Can you work these out from the model? Positions are in its coordinate system, mm. Face numbers are marked on the shaded views. A direction names the side the tool comes from. Round coordinates to 2 decimals unless told otherwise and drop trailing zeros. Write each loop counter-clockwise with the first axis right and the second up, starting at its lowest first coordinate (ties: lowest second). Pieces come first, ordered by that corner, then holes. Notation, with made-up numbers: (-13, 27.5) -> (17, 27.5) arc R13 cw to (17, 43.5) -> close; hole circle Ø1 at (-9.75, 58). An arc over 180 degrees is marked (long way). Write item = value, one per line. Start each with the question number.
1) I'm going to push flat-ended pins straight in: pin 1 (5 mm diameter, centred on y = 8.8, z = -53.6, fed in from -X); pin 2 (8 mm diameter, centred on x = -86, y = 8, fed in from -Z); pin 3 (2.5 mm diameter, centred on y = 34.5, z = -53.6, fed in from +X). Where does each tip first touch, or does it pass through?
2) If I drill on line 1 (Z direction, x = -7, y = 0.8); line 2 (Z direction, x = -66, y = 28); line 3 (X direction, y = 0.5, z = -90.6), over which ranges is the centre line in solid material (lowest first)?
3) Imagine slicing it at B-B, the plane z = -53.6. Please give me the cut outline in (x, y), then the cut area to 3 significant figures.
4) Thinking about a two-plate mould opening in Z: for the marked faces 3, 4 and 5, which applies, +Z half, -Z half, draft (parallel to the pull), parting line (faces both ways), or undercut?
5) Imagine slicing it at D-D, the plane x = -34. Please give me the cut outline in (y, z).
6) For the marked faces 1 and 2, which set-ups out of +Z, -Z, +X, -X, +Y, -Y let a thin tool reach every point of the face, with its end or its side?
7) Imagine slicing it at A-A, the plane z = -90.6. Please give me the cut outline in (x, y).
8) Imagine slicing it at C-C, the plane y = 8.8. State how many separate pieces and enclosed holes the cut face has, then the cut area to 3 significant figures.
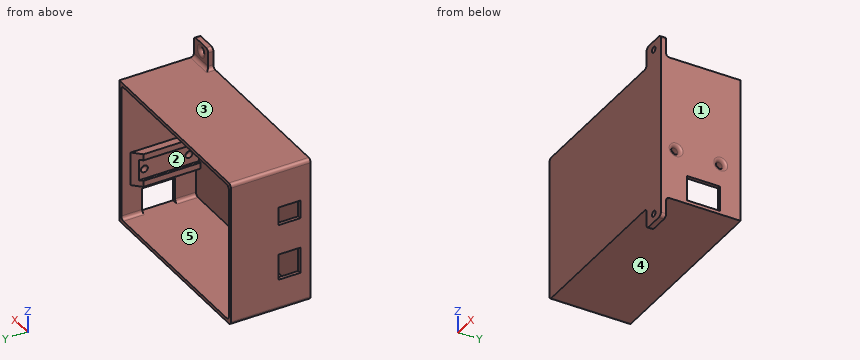
from build123d import *

# Parameters (mm, degrees)
BOSS_EXTRUDE1_DEPTH = 46
BOSS_EXTRUDE2_DEPTH = 3
BOSS_EXTRUDE3_DEPTH = 3
FILLET1_R           = 2
FILLET2_R           = 2
CUT_EXTRUDE5_REACH  = 154.825
SKETCH3_R           = 1.7
FILLET3_R           = 2
CUT_EXTRUDE6_DEPTH  = 43
SKETCH5_W           = 4.6
SKETCH5_H           = 19.4
BOSS_EXTRUDE4_DEPTH = 46
SKETCH6_W           = 4.6
SKETCH6_H           = 19.4
CUT_EXTRUDE8_DEPTH  = 5
SKETCH7_W           = 1.6
SKETCH7_H           = 12.2
CUT_EXTRUDE10_DEPTH = 38
CHAMFER1_SIZE       = 5
SKETCH8_R           = 2
CUT_EXTRUDE11_DEPTH = 34.5
FILLET4_R           = 2
SKETCH12_W          = 15
SKETCH12_H          = 12.6
SKETCH12_W_2        = 10.5
CUT_EXTRUDE13_DEPTH = 34.5
SKETCH14_W          = 14.5
SKETCH14_H          = 19
CUT_EXTRUDE14_DEPTH = 10


with BuildPart() as part:
    # Sketch2 → Boss-Extrude1 (new body)
    with BuildSketch(Plane(origin=(0, 0, 0), x_dir=(1, 0, 0), z_dir=(0, 1, 0))):
        with BuildLine():
            ThreePointArc((-110, 81.6), (-109.414213562, 83.014213562), (-108, 83.6))
            Line((-108, 83.6), (-16, 83.6))
            Line((-16, 83.6), (0, 83.6))
            Line((0, 83.6), (0, 0))
            Line((0, 0), (-16, 0))
            Line((-16, 0), (-108, 0))
            ThreePointArc((-108, 0), (-109.414213562, 0.585786438), (-110, 2))
            Line((-110, 2), (-110, 81.6))
        make_face()
    extrude(amount=BOSS_EXTRUDE1_DEPTH)

    # Sketch2<7> → Boss-Extrude2 (add)
    with BuildSketch(Plane(origin=(0, 0, 0), x_dir=(1, 0, 0), z_dir=(0, 1, 0))):
        with BuildLine():
            ThreePointArc((-16, 83.6), (-14.585786438, 84.185786438), (-14, 85.6))
            Line((-14, 85.6), (-14, 93.6))
            ThreePointArc((-14, 93.6), (-13.414213562, 95.014213562), (-12, 95.6))
            Line((-12, 95.6), (-2, 95.6))
            ThreePointArc((-2, 95.6), (-0.585786438, 95.014213562), (0, 93.6))
            Line((0, 93.6), (0, 83.6))
            Line((0, 83.6), (-16, 83.6))
        make_face()
    extrude(amount=BOSS_EXTRUDE2_DEPTH)

    # Sketch2<8> → Boss-Extrude3 (add)
    with BuildSketch(Plane(origin=(0, 0, 0), x_dir=(1, 0, 0), z_dir=(0, 1, 0))):
        with BuildLine():
            ThreePointArc((0, -10), (-0.585786438, -11.414213562), (-2, -12))
            Line((-2, -12), (-12, -12))
            ThreePointArc((-12, -12), (-13.414213562, -11.414213562), (-14, -10))
            Line((-14, -10), (-14, -2))
            ThreePointArc((-14, -2), (-14.585786438, -0.585786438), (-16, 0))
            Line((-16, 0), (0, 0))
            Line((0, 0), (0, -10))
        make_face()
    extrude(amount=BOSS_EXTRUDE3_DEPTH)

    # Fillet1
    fillet1_edges = [part.edges().sort_by_distance(p)[0] for p in [
        (-8, 3, -83.6),
    ]]
    fillet(fillet1_edges, radius=FILLET1_R)

    # Fillet2
    fillet2_edges = [part.edges().sort_by_distance(p)[0] for p in [
        (-8, 3, 0),
    ]]
    fillet(fillet2_edges, radius=FILLET2_R)

    # Sketch3 → Cut-Extrude5 (cut, up to next)
    with BuildSketch(Plane(origin=(0, 0, 0), x_dir=(1, 0, 0), z_dir=(0, 1, 0)), mode=Mode.PRIVATE) as cut_extrude5_sk1:
        with Locations(Location((-7, -7, 0), (0, 0, 270))):
            Circle(SKETCH3_R)
    cut_extrude5_tool1 = extrude(cut_extrude5_sk1.sketch, amount=CUT_EXTRUDE5_REACH, mode=Mode.PRIVATE) & part.part
    # Sketch3 → Cut-Extrude5 (cut, up to next)
    with BuildSketch(Plane(origin=(0, 0, 0), x_dir=(1, 0, 0), z_dir=(0, 1, 0)), mode=Mode.PRIVATE) as cut_extrude5_sk2:
        with Locations(Location((-7, 90.6, 0), (0, 0, 270))):
            Circle(SKETCH3_R)
    cut_extrude5_tool2 = extrude(cut_extrude5_sk2.sketch, amount=CUT_EXTRUDE5_REACH, mode=Mode.PRIVATE) & part.part
    add(cut_extrude5_tool1.solids().sort_by_distance((-7, 0, 7))[0], mode=Mode.SUBTRACT)
    add(cut_extrude5_tool2.solids().sort_by_distance((-7, 0, -90.6))[0], mode=Mode.SUBTRACT)

    # Fillet3
    fillet3_edges = [part.edges().sort_by_distance(p)[0] for p in [
        (-7, 3, -92.3),
        (-7, 3, 5.3),
    ]]
    fillet(fillet3_edges, radius=FILLET3_R)

    # Sketch4 → Cut-Extrude6 (cut)
    with BuildSketch(Plane(origin=(0, 46, 0), x_dir=(1, 0, 0), z_dir=(0, 1, 0))):
        with BuildLine():
            Line((-106, 81.6), (-4, 81.6))
            ThreePointArc((-4, 81.6), (-2.585786438, 81.014213562), (-2, 79.6))
            Line((-2, 79.6), (-2, 4))
            ThreePointArc((-2, 4), (-2.585786438, 2.585786438), (-4, 2))
            Line((-4, 2), (-106, 2))
            ThreePointArc((-106, 2), (-107.414213562, 2.585786438), (-108, 4))
            Line((-108, 4), (-108, 79.6))
            ThreePointArc((-108, 79.6), (-107.414213562, 81.014213562), (-106, 81.6))
        make_face()
    extrude(amount=-CUT_EXTRUDE6_DEPTH, mode=Mode.SUBTRACT)

    # Sketch5 → Boss-Extrude4 (add)
    with BuildSketch(Plane(origin=(0, 0, 0), x_dir=(1, 0, 0), z_dir=(0, 1, 0))):
        with Locations((-4.3, 53.3)):
            Rectangle(SKETCH5_W, SKETCH5_H)
    extrude(amount=BOSS_EXTRUDE4_DEPTH)

    # Sketch6 → Cut-Extrude8 (cut)
    with BuildSketch(Plane(origin=(0, 46, 0), x_dir=(1, 0, 0), z_dir=(0, 1, 0))):
        with Locations((-4.3, 53.3)):
            Rectangle(SKETCH6_W, SKETCH6_H)
    extrude(amount=-CUT_EXTRUDE8_DEPTH, mode=Mode.SUBTRACT)

    # Sketch7 → Cut-Extrude10 (cut)
    with BuildSketch(Plane(origin=(0, 41, 0), x_dir=(1, 0, 0), z_dir=(0, 1, 0))):
        with Locations((-5.8, 53.3)):
            Rectangle(SKETCH7_W, SKETCH7_H)
    extrude(amount=-CUT_EXTRUDE10_DEPTH, mode=Mode.SUBTRACT)

    # Chamfer1
    # the kernel refuses this chamfer: 5 mm, written as the material it takes off along each edge
    with BuildSketch(Plane(origin=(-6.6, 41, -46.54158506), x_dir=(0.9996219169112968, 0.027495876610586317, 0), z_dir=(0, 0, -1))) as chamfer1_piece_1_section:
        Polygon((CHAMFER1_SIZE * 0.999621916911, CHAMFER1_SIZE * 0.0274958766106), (-CHAMFER1_SIZE * 0.0274958766106, CHAMFER1_SIZE * 0.999621916911), (0, 0), align=None)
    chamfer1_piece_1 = extrude(amount=29.31682988, mode=Mode.PRIVATE)
    chamfer1_piece_1 = split(chamfer1_piece_1, bisect_by=Plane(origin=(-2, 39.327890325, -61.2), z_dir=(-1, 0, 0)), keep=Keep.TOP, mode=Mode.PRIVATE)
    add(chamfer1_piece_1, mode=Mode.SUBTRACT)
    with BuildSketch(Plane(origin=(-6.6, 41, -30.74158506), x_dir=(0.9996219169112968, 0.027495876610586317, 0), z_dir=(0, 0, -1))) as chamfer1_piece_2_section:
        Polygon((CHAMFER1_SIZE * 0.999621916911, CHAMFER1_SIZE * 0.0274958766106), (-CHAMFER1_SIZE * 0.0274958766106, CHAMFER1_SIZE * 0.999621916911), (0, 0), align=None)
    chamfer1_piece_2 = extrude(amount=29.31682988, mode=Mode.PRIVATE)
    chamfer1_piece_2 = split(chamfer1_piece_2, bisect_by=Plane(origin=(-2, 39.327890325, -45.4), z_dir=(-1, 0, 0)), keep=Keep.TOP, mode=Mode.PRIVATE)
    add(chamfer1_piece_2, mode=Mode.SUBTRACT)

    # Sketch8 → Cut-Extrude11 (cut)
    with BuildSketch(Plane(origin=(0, 0, 0), x_dir=(0, 0, -1), z_dir=(1, 0, 0))):
        with Locations((53.6, 8.8)):
            Circle(SKETCH8_R)
        with Locations((53.6, 34.5)):
            Circle(SKETCH8_R)
    extrude(amount=-CUT_EXTRUDE11_DEPTH, mode=Mode.SUBTRACT)

    # Fillet4
    fillet4_edges = [part.edges().sort_by_distance(p)[0] for p in [
        (0, 8.8, -51.6),
        (0, 34.5, -51.6),
    ]]
    fillet(fillet4_edges, radius=FILLET4_R)

    # Sketch12 → Cut-Extrude13 (cut)
    with BuildSketch(Plane.ZY.offset(110)):
        with Locations((-58.05, 12.3)):
            Rectangle(SKETCH12_W, SKETCH12_H)
        with Locations((-27.8, 12.3)):
            Rectangle(SKETCH12_W_2, SKETCH12_H)
    extrude(amount=-CUT_EXTRUDE13_DEPTH, mode=Mode.SUBTRACT)

    # Sketch14 → Cut-Extrude14 (cut)
    with BuildSketch(Plane(origin=(0, 0, 0), x_dir=(0, 0, -1), z_dir=(1, 0, 0))):
        with Locations((74.35, 24.5)):
            Rectangle(SKETCH14_W, SKETCH14_H)
    extrude(amount=-CUT_EXTRUDE14_DEPTH, mode=Mode.SUBTRACT)


solid = part.part
Reported:
q1.pin_1 = -5
q1.pin_2 = -83.6
q1.pin_3 = -108
q2.line_1 = -95.6 to -92.3, -88.9 to 5.3, 8.7 to 12
q2.line_2 = -83.6 to -81.6, -2 to 0
q2.line_3 = -14 to -8.7, -5.3 to 0
q3.outline = (-110, 0) -> (0, 0) -> (0, 4.8) arc R2 ccw to (-2, 6.8) -> (-5, 6.8) -> (-5, 3) -> (-108, 3) -> (-108, 6) -> (-110, 6) -> close; (-110, 18.6) -> (-108, 18.6) -> (-108, 46) -> (-110, 46) -> close; (-5, 10.8) -> (-2, 10.8) arc R2 ccw to (0, 12.8) -> (0, 30.5) arc R2 ccw to (-2, 32.5) -> (-5, 32.5) -> close; (-5, 36.5) -> (-2, 36.5) arc R2 ccw to (0, 38.5) -> (0, 46) -> (-2, 46) -> (-2, 40.6) -> (-5, 37.6) -> close
q3.area = 542 mm²
q4.face_3 = +Z half
q4.face_4 = -Z half
q4.face_5 = undercut
q5.outline = (0, -83.6) -> (46, -83.6) -> (46, -81.6) -> (3, -81.6) -> (3, -2) -> (46, -2) -> (46, 0) -> (0, 0) -> close
q6.face_1 = +Z, -Z, +X, +Y, -Y
q6.face_2 = +Y
q7.outline = (-14, 0) -> (-8.7, 0) -> (-8.7, 1) arc R2 ccw to (-10.7, 3) -> (-14, 3) -> close; (-5.3, 0) -> (0, 0) -> (0, 3) -> (-3.3, 3) arc R2 ccw to (-5.3, 1) -> close
q8.separate_pieces = 3
q8.enclosed_holes = 0
q8.area = 757 mm²
